```python
from build123d import *

# Parameters (mm, degrees)
SKETCH1_W               = 50.8
SKETCH1_H               = 40.64
BOSS_EXTRUDE1_DEPTH     = 12.7
CUT_EXTRUDE1_DEPTH      = 67.283780822
CUT_EXTRUDE1_DEPTH_BACK = 67.283780822
CUT_EXTRUDE2_DEPTH      = 67.283780822
CUT_EXTRUDE2_DEPTH_BACK = 67.283780822
SKETCH3_R               = 3.429
FILLET1_R               = 6.35


with BuildPart() as part:
    # Sketch1 → Boss-Extrude1 (new body)
    with BuildSketch(Plane(origin=(0, 0, 0), x_dir=(1, 0, 0), z_dir=(0, 1, 0))):
        with Locations((25.4, 20.32)):
            Rectangle(SKETCH1_W, SKETCH1_H)
    extrude(amount=BOSS_EXTRUDE1_DEPTH)

    # Sketch2 → Cut-Extrude1 (cut, two sides: drawn at the far end of the back side and taken through both)
    with BuildSketch(Plane.XY.offset(-CUT_EXTRUDE1_DEPTH_BACK)):
        with BuildLine():
            Line((33.909, 12.7), (25.4, 12.7))
            Line((25.4, 12.7), (25.4, 4.448908618))
            ThreePointArc((25.4, 4.448908618), (31.400662292, 6.773711322), (33.909, 12.7))
        make_face()
        with BuildLine():
            Line((25.4, 4.448908618), (25.4, 12.7))
            Line((25.4, 12.7), (17.399, 12.7))
            ThreePointArc((17.399, 12.7), (19.727711322, 6.953337708), (25.4, 4.448908618))
        make_face()
        with BuildLine():
            Line((33.909, 12.7), (25.4, 12.7))
            Line((25.4, 12.7), (25.4, 4.448908618))
            ThreePointArc((25.4, 4.448908618), (31.400662292, 6.773711322), (33.909, 12.7))
        make_face()
        with BuildLine():
            Line((25.4, 4.448908618), (25.4, 12.7))
            Line((25.4, 12.7), (17.399, 12.7))
            ThreePointArc((17.399, 12.7), (19.727711322, 6.953337708), (25.4, 4.448908618))
        make_face()
    extrude(amount=CUT_EXTRUDE1_DEPTH + CUT_EXTRUDE1_DEPTH_BACK, mode=Mode.SUBTRACT)

    # Sketch3 → Cut-Extrude2 (cut, two sides: drawn at the far end of the back side and taken through both)
    with BuildSketch(Plane(origin=(0, 12.7, 0), x_dir=(1, 0, 0), z_dir=(0, 1, 0)).offset(-CUT_EXTRUDE2_DEPTH_BACK)):
        with Locations(Location((8.6995, 10.16, 0), (0, 0, 270))):
            Circle(SKETCH3_R)
        with Locations(Location((42.2275, 10.16, 0), (0, 0, 270))):
            Circle(SKETCH3_R)
        with Locations(Location((42.2275, 30.48, 0), (0, 0, 270))):
            Circle(SKETCH3_R)
        with Locations(Location((8.6995, 30.48, 0), (0, 0, 270))):
            Circle(SKETCH3_R)
    extrude(amount=CUT_EXTRUDE2_DEPTH + CUT_EXTRUDE2_DEPTH_BACK, mode=Mode.SUBTRACT)

    # Fillet1
    fillet1_edges = [part.edges().sort_by_distance(p)[0] for p in [
        (0, 6.35, -40.64),
        (50.8, 6.35, -40.64),
        (50.8, 6.35, 0),
        (0, 6.35, 0),
    ]]
    fillet(fillet1_edges, radius=FILLET1_R)


solid = part.part
```
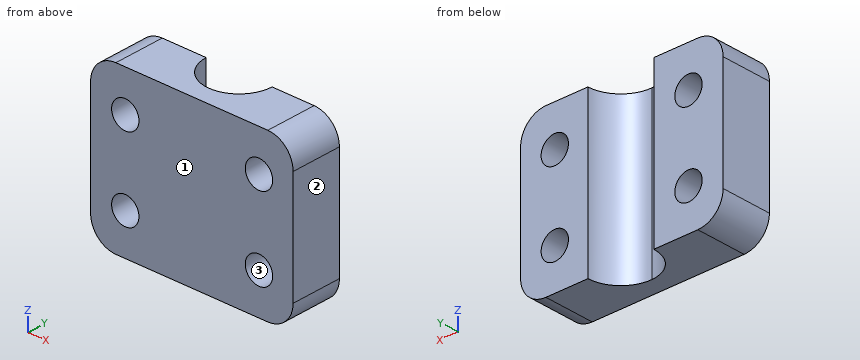
Geometry: final body of the model. Coordinates: model frame, mm. Face numbers are marked on the shaded views. Round coordinates to 2 decimals unless told otherwise and drop trailing zeros. Order: outer loops, then holes, each group sorted by start corner. A loop starts at its lowest first (then second) coordinate and runs counter-clockwise, first axis right, second up. Notation, with made-up numbers: (-37, -39.5) -> (-20, -39.5) arc R36 ccw to (-20, -0.5) -> close; hole circle Ø5 at (63, 0.5). An arc over 180 degrees is marked (long way). Write each question's results on one line, items separated by ' | '.
Q1. Section query D-D (z = -23.5). Output: boundary loops of the cut face in (x, y) (3 decimals).
Response values:
outline: (0, 0) -> (50.8, 0) -> (50.8, 12.7) -> (33.909, 12.7) arc R8.255 cw to (17.399, 12.7) -> (0, 12.7) -> close
Q2. Section query C-C (y = 1.5). Output: boundary loops of the cut face in (x, z).
Response values:
outline: (0, -34.29) arc R6.35 ccw to (6.35, -40.64) -> (44.45, -40.64) arc R6.35 ccw to (50.8, -34.29) -> (50.8, -6.35) arc R6.35 ccw to (44.45, 0) -> (6.35, 0) arc R6.35 ccw to (0, -6.35) -> close; hole circle Ø6.86 at (8.7, -30.48); hole circle Ø6.86 at (8.7, -10.16); hole circle Ø6.86 at (42.23, -30.48); hole circle Ø6.86 at (42.23, -10.16)
Q3. Pin query (flat end, axial travel): pin 1 Ø3 at (x, z) = (14.5, -30) entering from -Y. Return the tip coordinate at first contact, or that it passes through.
Response values:
pin 1: y = 0
Q4. Section query B-B (y = 6.25). Output: boundary loops of the cut face in (x, z), and give its area (3 significant figures).
Response values:
outline: (0, -34.29) arc R6.35 ccw to (6.35, -40.64) -> (20.5, -40.64) -> (20.5, 0) -> (6.35, 0) arc R6.35 ccw to (0, -6.35) -> close; (30.81, -40.64) -> (44.45, -40.64) arc R6.35 ccw to (50.8, -34.29) -> (50.8, -6.35) arc R6.35 ccw to (44.45, 0) -> (30.81, 0) -> close; hole circle Ø6.86 at (8.7, -30.48); hole circle Ø6.86 at (8.7, -10.16); hole circle Ø6.86 at (42.23, -30.48); hole circle Ø6.86 at (42.23, -10.16) | area: 1,460 mm²
Q5. Section query A-A (z = -30.48). Output: boundary loops of the cut face in (x, y) (1 decimal).
Response values:
outline: (0, 0) -> (5.3, 0) -> (5.3, 12.7) -> (0, 12.7) -> close; (12.1, 0) -> (38.8, 0) -> (38.8, 12.7) -> (33.9, 12.7) arc R8.3 cw to (17.4, 12.7) -> (12.1, 12.7) -> close; (45.7, 0) -> (50.8, 0) -> (50.8, 12.7) -> (45.7, 12.7) -> close
Q6. Pull-direction query (X, two-part tool) for the marked faces 1, 2 and 3; classes: released by +X, released by -X, zero draft, split by the parting line, or undercut.
Response values:
face 1: zero draft | face 2: released by +X | face 3: undercut
Q7. Ray query, line 1 along X through (y, z) = (1.75, -28); line 2 along Z through (x, y) = (6.5, 7); line 3 along X through (y, z) = (6.25, -10.16). Return the intervals inside material, ascending.
Response values:
line 1: 0 to 6.33, 11.07 to 39.86, 44.6 to 50.8 | line 2: -40.64 to -33.11, -27.85 to -12.79, -7.53 to 0 | line 3: 0 to 5.27, 12.13 to 20.5, 30.81 to 38.8, 45.66 to 50.8
